```python
from build123d import *

# Parameters (mm, degrees)
F0_W     = 60
F0_H     = 15
F1_DEPTH = 100
F2_W     = 40
F2_H     = 10
F3_DEPTH = 30
F4_W     = 10
F4_H     = 30
F5_DEPTH = 25


with BuildPart() as f1:
    # F0 (on Front) → F1 (new body)
    with BuildSketch(Plane.XZ):
        Rectangle(F0_W, F0_H)
    extrude(amount=-F1_DEPTH)

    # F2 (on face) → F3 (cut)
    with BuildSketch(Plane.XZ):
        Rectangle(F2_W, F2_H)
    extrude(amount=-F3_DEPTH, mode=Mode.SUBTRACT)

    # F4 (on face) → F5 (cut)
    with BuildSketch(Plane.XY.offset(-5)):
        with Locations((-1, 15)):
            Rectangle(F4_W, F4_H)
    extrude(amount=-F5_DEPTH, mode=Mode.SUBTRACT)


solid = f1.part
```
Verification items for the finished model (mm, model axes). A direction names the side the tool comes from. Give positions to 0.01 mm unless a question says otherwise; leave off trailing zeros. Write each loop counter-clockwise with the first axis right and the second up, starting at its lowest first coordinate (ties: lowest second). Pieces come first, ordered by that corner, then holes. Notation, with made-up numbers: M 83.5,88 L 134.5,88 A26 ccw 134.5,109 Z; hole C 7.5,80.5 d8. An arc over 180 degrees is marked long. One line per question, with ' | ' between items.
1) Section check B-B on x = 9. Enter the section's corners in (y, z).
Result:
outline: M 0,-7.5 L 100,-7.5 L 100,7.5 L 0,7.5 L 0,5 L 30,5 L 30,-5 L 0,-5 Z
2) Mould release check, pull along X, two halves, no side actions. Record for faces 1 (the flat face through (12, 15, -5)), 2 (the flat face through (0, 0, 7)), 3 (the flat face through (-30, 49, 0)): released by +X, released by -X, zero draft, split by the parting line, or undercut.
Result:
face 1: undercut | face 2: zero draft | face 3: released by -X
3) Thickness scan on line 1 along Z through (x, y) = (-17, 17); line 2 along X through (y, z) = (26.5, -4.5); line 3 along Y through (x, z) = (4, 3). Record the ranges inside material, lowest first. Write a range as [from, to].
Result:
line 1: z = [-7.5, -5], [5, 7.5] | line 2: x = [-30, -20], [20, 30] | line 3: y = [30, 100]
4) Section check A-A on z = 3.5. Enter the section's corners in (x, y), plus the area to 3 significant figures.
Result:
outline: M -30,0 L -20,0 L -20,30 L 20,30 L 20,0 L 30,0 L 30,100 L -30,100 Z | area: 4,800 mm2
5) Section check C-C on x = -5. Enter the section's corners in (y, z).
Result:
outline: M 0,5 L 30,5 L 30,-7.5 L 100,-7.5 L 100,7.5 L 0,7.5 Z
6) Gauge pin test, flat end, axial feed: pin 1 Ø4 at (x, z) = (10, -1.5) entering from -Y. Record the tip position at first contact, or that the pin passes through.
Result:
pin 1: stops at y = 30
7) Set-up check for faces 4 (the flat face through (-6, 15, -6)), 5 (the flat face through (30, 49, 0)), 6 (the flat face through (-20, 15, 0)): record each of +Z, -Z, +X, -X, +Y, -Y from which the full face is reachable in a straight line by a thin tool's end or side.
Result:
face 4: -Z, -Y | face 5: +Z, -Z, +X, +Y, -Y | face 6: -Y
